Autodesk Fusion 360 part; units mm, degrees
sketch "Esquisse1" plane through (0, 0, 0) normal (0, 0, 1) x (1, 0, 0)
  circle A0 centre (0, 0) radius 4.2
  circle A1 centre (0, 0) radius 7.5
  dimension "d1" = 8.4
  dimension "d2" = 15
extrude "Extrusion1" add sketch "Esquisse1" along normal blind 8
hole "Perçage1" at (0, -7.5, 4) direction (0, 1, 0) diameter 3.5 depth 15 tip angle 180 counterbore diameter 6 counterbore depth 2
ref_plane "Plan de construction1" through (0, 7.5, 0) normal (0, 1, 0) x (0, 0, 1)
sketch "Esquisse2" plane through (0, 7.5, 0) normal (0, 1, 0) x (1, 0, 0)
  line L0 (-2.9935, -2.2568) -> (-3.0064, -5.7209)
  line L1 (-3.0064, -5.7209) -> (-0.0129, -7.4641)
  line L2 (-0.0129, -7.4641) -> (2.9935, -5.7432)
  line L3 (2.9935, -5.7432) -> (3.0064, -2.2791)
  line L4 (3.0064, -2.2791) -> (0.0129, -0.5359)
  line L5 (0.0129, -0.5359) -> (-2.9935, -2.2568)
  point P0 (0, -4)
  dimension "d12" = 3
extrude "Extrusion2" cut sketch "Esquisse2" against normal blind 2
chamfer "Chanfrein1" distance 0.5 angle 45 1 edges at (-3.9158, 1.5188, 8)
chamfer "Chanfrein2" distance 0.5 angle 45 1 edges at (-6.9925, -2.7121, 8)
For this review, take the finished solid that the model builds, in its own axes (mm). A direction names the side the tool comes from. Give positions to 0.01 mm unless a question says otherwise; leave off trailing zeros. Write each loop counter-clockwise with the first axis right and the second up, starting at its lowest first coordinate (ties: lowest second). Pieces come first, ordered by that corner, then holes.
Item 1: Take a section at D-D (x = -0.5). Give the number of separate pieces and of enclosed holes in the cut face, and give its area (3 significant figures).
Item 2: Machinability: for faces 4 (the face through (1.3, 5.5, 5.5)), 5 (the face through (2, -5.5, 4)), 6 (the face through (6.93, 2.87, 3.7)), which of the approach directions +Z, -Z, +X, -X, +Y, -Y give a long, thin tool a straight path to every point of the face, cutting with its end or side? Answer none if there is none.
Item 3: Take a section at A-A (y = 0). Give the boundary of the cut face in (x, z), and give its area (3 significant figures).
Item 4: The part is to be moulded in two halves that separate along Z. For faces 1 (the face through (3.2, -3.2, 0)), 2 (the face through (1.5, 6.5, 6.6)), 3 (the face through (1, -5, 8)), say which applies: +Z half, -Z half, draft (parallel to the pull), parting line (faces both ways), or undercut.
Item 5: Wall thickness on probe 1 along Z at (x, y) = (0, -6.2); probe 2 along X at (y, z) = (-5.1, 4); probe 3 along Y at (x, z) = (0.25, 6.5): over which ranges is each line inside the solid? List them lowest first.
Item 6: Insertion check: P1, Ø2, axis at x = -5, z = 6.5, coming from the +Y side; P2, Ø1.8, axis at x = 0, z = 3, coming from the +Y side; P3, Ø1.5, axis at y = 5, z = 3.5, coming from the -X side. Each pin has a flat end and moves straight along its axis. Give the tip position at first contact, or say it passes through.
Item 7: Take a section at C-C (z = 7.75). Give the boundary of the cut face in (x, y).
Item 8: Take a section at B-B (z = 4). Give the boundary of the cut face in (x, y).
Established:
1. separate pieces: 4
1. enclosed holes: 0
1. area: 19.3 mm2
2. face 4: +Y
2. face 5: -Y
2. face 6: +Z, -Z
3. outline: (-7.5, 0) - (-4.2, 0) - (-4.2, 7.5) - (-4.7, 8) - (-7, 8) - (-7.5, 7.5) - close; (4.2, 0) - (7.5, 0) - (7.5, 7.5) - (7, 8) - (4.7, 8) - (4.2, 7.5) - close
3. area: 52.3 mm2
4. face 1: -Z half
4. face 2: undercut
4. face 3: +Z half
5. probe 1: z = 0 to 1, 7 to 8
5. probe 2: x = -5.5 to -1.75, 1.75 to 5.5
5. probe 3: y = -5.5 to -4.19, 4.19 to 5.5
6. P1: stops at y = 6.34
6. P2: stops at y = 5.5
6. P3: stops at x = -6.18
7. outline: circle Ø14.5 at (0, 0); hole circle Ø8.9 at (0, 0)
8. outline: (-3, -6.87) - (-3, -5.5) - (-1.75, -5.5) - (-1.75, -3.82) arc R4.2 cw to (-1.75, 3.82) - (-1.75, 5.5) - (-3, 5.5) - (-3, 6.87) arc R7.5 ccw to start; (1.75, -5.5) - (3, -5.5) - (3, -6.87) arc R7.5 ccw to (3, 6.87) - (3, 5.5) - (1.75, 5.5) - (1.75, 3.82) arc R4.2 cw to (1.75, -3.82) - close
